```python
from build123d import *

# Parameters (mm, degrees)
SKETCH_1_R      = 14.2
EXTRUDE_1_DEPTH = 4.1
EXTRUDE_2_DEPTH = 1
SKETCH_2_4_R    = 7.65
EXTRUDE_3_DEPTH = 4.8


with BuildPart() as part:
    # Sketch 1 → Extrude 1 (new body)
    with BuildSketch(Plane(origin=(0, 0, 0), x_dir=(1, 0, 0), z_dir=(0, 1, 0))):
        with Locations(Location((0, 0, 0), (0, 0, 270))):
            Circle(SKETCH_1_R)
    extrude(amount=EXTRUDE_1_DEPTH)

    # Sketch 2 → Extrude 2 (add)
    with BuildSketch(Plane(origin=(0, 4.1, 0), x_dir=(1, 0, 0), z_dir=(0, 1, 0))):
        with BuildLine():
            ThreePointArc((7.106423151, -7.106423151), (0, 10.05), (-7.106423151, -7.106423151))
            Line((-7.106423151, -7.106423151), (-10.040916293, -10.040916293))
            ThreePointArc((-10.040916293, -10.040916293), (0, -14.2), (10.040916293, -10.040916293))
            Line((10.040916293, -10.040916293), (7.106423151, -7.106423151))
        make_face()
    extrude(amount=EXTRUDE_2_DEPTH)

    # Sketch 2_4 → Extrude 3 (add)
    with BuildSketch(Plane(origin=(0, 4.1, 0), x_dir=(1, 0, 0), z_dir=(0, 1, 0))):
        with Locations(Location((0, 0, 0), (0, 0, 270))):
            Circle(SKETCH_2_4_R)
    extrude(amount=EXTRUDE_3_DEPTH)


solid = part.part
```
Design review of the part built by this model. Coordinates are the model's own, in mm. A direction names the side the tool comes from. Coordinates: 2 decimals unless noted, no trailing zeros. Loops run counter-clockwise (first coordinate to the right, second up) from the corner with the lowest first, then second, coordinate; pieces in that order, holes last. Notation, with made-up numbers: (14, 82.5) -> (44, 82.5) arc R23 cw to (44, 96.5) -> close; hole circle Ø2 at (44.5, 59.5). An arc over 180 degrees is marked (long way). Answer as a JSON object with one key per item and string values.
Q1. Take a section at A-A on z = 0. Give the boundary of the cut face in (x, y), plus the area to 3 significant figures.
Answer block:
{"outline": "(-14.2, 0) -> (14.2, 0) -> (14.2, 4.1) -> (10.05, 4.1) -> (10.05, 5.1) -> (7.65, 5.1) -> (7.65, 8.9) -> (-7.65, 8.9) -> (-7.65, 5.1) -> (-10.05, 5.1) -> (-10.05, 4.1) -> (-14.2, 4.1) -> close", "area": "195 mm^2"}
Q2. The part is to be moulded in two halves that separate along Z. For faces 1 (the flat face through (8.6, 4.6, 8.6)), 2 (the flat face through (-5, 5.1, 7)), 3 (the cylindrical face through (-4.655, 6.973, -6.071)), say which applies: +Z half, -Z half, draft (parallel to the pull), parting line (faces both ways), or undercut.
Answer block:
{"face 1": "undercut", "face 2": "draft", "face 3": "parting line"}
Q3. To check wall thickness, follow L1, parallel to Y at x = 8, z = 11; L2, parallel to Y at x = 11.75, z = 0.5; L3, parallel to Z at x = 1.5, y = 1. State the ranges of each line that lie inside material, in increasing order.
Answer block:
{"L1": "y = 0 to 5.1", "L2": "y = 0 to 4.1", "L3": "z = -14.12 to 14.12"}
Q4. Take a section at C-C on y = 5.5. Give the boundary of the cut face in (x, z).
Answer block:
{"outline": "circle Ø15.3 at (0, 0)"}
Q5. Clearance check with flat-ended pins moving along their axes: pin 1 Ø3 at (x, z) = (-10.5, 9) entering from +Y; pin 2 Ø4 at (y, z) = (4, -9.5) entering from +X; pin 3 Ø1.5 at (x, y) = (2, 3) entering from +Z. State where each tip first meets the part, or that it passes through.
Answer block:
{"pin 1": "stops at y = 5.1", "pin 2": "stops at x = 12.06", "pin 3": "stops at z = 14.14"}
Q6. Tool access review of faces 4 (the flat face through (0, 8.9, 0)), 5 (the flat face through (-8.6, 4.6, 8.6)), 6 (the cylindrical face through (0.331, 4.593, -10.045)): name each direction out of +Z, -Z, +X, -X, +Y, -Y from which nothing blocks a thin tool from reaching the whole face with its end or side.
Answer block:
{"face 4": "+Z, -Z, +X, -X, +Y", "face 5": "-X, +Y", "face 6": "+Y"}
Q7. Take a section at B-B on x = 0. Give the boundary of the cut face in (y, z).
Answer block:
{"outline": "(0, -14.2) -> (4.1, -14.2) -> (4.1, -10.05) -> (5.1, -10.05) -> (5.1, -7.65) -> (8.9, -7.65) -> (8.9, 7.65) -> (5.1, 7.65) -> (5.1, 14.2) -> (0, 14.2) -> close"}
Q8. Take a section at D-D on z = -4. Give the boundary of the cut face in (x, y).
Answer block:
{"outline": "(-13.62, 0) -> (13.62, 0) -> (13.62, 4.1) -> (9.22, 4.1) -> (9.22, 5.1) -> (6.52, 5.1) -> (6.52, 8.9) -> (-6.52, 8.9) -> (-6.52, 5.1) -> (-9.22, 5.1) -> (-9.22, 4.1) -> (-13.62, 4.1) -> close"}
